```python
from build123d import *

# Parameters (mm, degrees)
SKETCH_1_R      = 15
SKETCH_1_R_2    = 1
EXTRUDE_1_DEPTH = 2
EXTRUDE_2_DEPTH = 1
SKETCH_4_R      = 10.5
SKETCH_4_R_2    = 0.75
EXTRUDE_3_DEPTH = 2
SKETCH_5_R      = 10.5
SKETCH_5_R_2    = 0.75
EXTRUDE_4_DEPTH = 2
EXTRUDE_5_DEPTH = 1
SKETCH_7_R      = 10.5
SKETCH_7_R_2    = 0.75
EXTRUDE_6_DEPTH = 2
SKETCH_8_R      = 10.5
SKETCH_8_R_2    = 0.75
EXTRUDE_7_DEPTH = 2


with BuildPart() as part:
    # 草图1 → 凸台-拉伸1 (new body)
    with BuildSketch(Plane(origin=(0, 0, 0), x_dir=(1, 0, 0), z_dir=(0, 1, 0))):
        with Locations(Location((0, 0, 0), (0, 0, 270))):
            Circle(SKETCH_1_R)
        with Locations(Location((7.778174593, 7.778174593, 0), (0, 0, 270))):
            Circle(SKETCH_1_R_2, mode=Mode.SUBTRACT)
        with Locations(Location((-7.778174593, 7.778174593, 0), (0, 0, 270))):
            Circle(SKETCH_1_R_2, mode=Mode.SUBTRACT)
        with Locations(Location((-7.778174593, -7.778174593, 0), (0, 0, 270))):
            Circle(SKETCH_1_R_2, mode=Mode.SUBTRACT)
        with Locations(Location((7.778174593, -7.778174593, 0), (0, 0, 270))):
            Circle(SKETCH_1_R_2, mode=Mode.SUBTRACT)
    extrude(amount=EXTRUDE_1_DEPTH)

    # 草图2 → 旋转1 (revolve)
    with BuildSketch(Plane(origin=(0, 0, 0), x_dir=(0, 0, -1), z_dir=(1, 0, 0))):
        with BuildLine():
            Line((0, 2), (0, 7))
            ThreePointArc((0, 7), (3.535533906, 5.535533906), (5, 2))
            Line((5, 2), (0, 2))
        make_face()
    revolve(axis=Axis((0, 2, 0), (0, 1, 0)))

    # 草图3 → 凸台-拉伸2 (add, symmetric)
    with BuildSketch(Plane.XY):
        Polygon((0, 2), (24.148145657, 8.470476128), (16.420739047, 8.470476128), (0, 4.070552361), (0, 4.828427125), (-28.991378029, 33.819805153), (-31.819805153, 33.819805153), align=None)
    extrude(amount=EXTRUDE_2_DEPTH, both=True)

    # 草图4 → 凸台-拉伸3 (add)
    with BuildSketch(Plane(origin=(0, 8.470476128, 0), x_dir=(1, 0, 0), z_dir=(0, 1, 0))):
        with Locations(Location((29.148145657, 0, 0), (0, 0, 174.5349762))):
            Circle(SKETCH_4_R)
        with Locations(Location((29.148145657, 0, 0), (0, 0, 270))):
            Circle(SKETCH_4_R_2, mode=Mode.SUBTRACT)
    extrude(amount=EXTRUDE_3_DEPTH)

    # 草图5 → 凸台-拉伸4 (add)
    with BuildSketch(Plane(origin=(0, 33.819805153, 0), x_dir=(1, 0, 0), z_dir=(0, 1, 0))):
        with Locations(Location((-36.819805153, 0, 0), (0, 0, 270))):
            Circle(SKETCH_5_R)
        with Locations(Location((-36.819805153, 0, 0), (0, 0, 270))):
            Circle(SKETCH_5_R_2, mode=Mode.SUBTRACT)
    extrude(amount=EXTRUDE_4_DEPTH)

    # 草图6 → 凸台-拉伸5 (add, symmetric)
    with BuildSketch(Plane(origin=(0, 0, 0), x_dir=(0, 0, -1), z_dir=(1, 0, 0))):
        Polygon((0, 2), (30.310889132, 19.5), (26.310889132, 19.5), (0, 4.309401077), (0, 6), (-20.190598923, 40.97114317), (-22.5, 40.97114317), align=None)
    extrude(amount=EXTRUDE_5_DEPTH, both=True)

    # 草图7 → 凸台-拉伸6 (add)
    with BuildSketch(Plane(origin=(0, 19.5, 0), x_dir=(1, 0, 0), z_dir=(0, 1, 0))):
        with Locations(Location((0, 35.310889132, 0), (0, 0, 270))):
            Circle(SKETCH_7_R)
        with Locations(Location((0, 35.310889132, 0), (0, 0, 270))):
            Circle(SKETCH_7_R_2, mode=Mode.SUBTRACT)
    extrude(amount=EXTRUDE_6_DEPTH)

    # 草图8 → 凸台-拉伸7 (add)
    with BuildSketch(Plane(origin=(0, 40.97114317, 0), x_dir=(1, 0, 0), z_dir=(0, 1, 0))):
        with Locations(Location((0, -27.5, 0), (0, 0, 270))):
            Circle(SKETCH_8_R)
        with Locations(Location((0, -27.5, 0), (0, 0, 270))):
            Circle(SKETCH_8_R_2, mode=Mode.SUBTRACT)
    extrude(amount=EXTRUDE_7_DEPTH)


solid = part.part
```
Work out the finished part from the listing and answer in its coordinate system (mm). A direction names the side the tool comes from. Give positions to 0.01 mm unless a question says otherwise; leave off trailing zeros. Write each loop counter-clockwise with the first axis right and the second up, starting at its lowest first coordinate (ties: lowest second). Pieces come first, ordered by that corner, then holes.
(1) The part is cut by section D-D on x = 33. Write down the section's boundary in (y, z), plus the area to 3 significant figures.
Final values:
outline: (8.47, -9.77) - (10.47, -9.77) - (10.47, 9.77) - (8.47, 9.77) - close
area: 39.1 mm2
(2) The part is cut by section B-B on y = 32.5. Write down the section's boundary in (x, z), plus the area to 3 significant figures.
Final values:
outline: (-30.5, -1) - (-27.67, -1) - (-27.67, 1) - (-30.5, 1) - close; (-1, 15.3) - (1, 15.3) - (1, 17.61) - (-1, 17.61) - close
area: 10.3 mm2
(3) Flat-ended cylindrical pins translate along their axes: pin 1 Ø8 at (y, z) = (16.5, -18.5) entering from -X; pin 2 Ø2 at (x, z) = (-8.5, -32) entering from +Y; pin 3 Ø23 at (x, z) = (-38, -2.5) entering from +Y; pin 4 Ø2.5 at (x, z) = (-7.78, 7.78) entering from -Y. Find the tip coordinate at first contact, or state that the pin passes through.
Final values:
pin 1: stops at x = -1
pin 2: stops at y = 21.5
pin 3: stops at y = 35.82
pin 4: stops at y = 0
(4) The part is cut by section C-C on z = 13. Write down the section's boundary in (x, y), plus the area to 3 significant figures.
Final values:
outline: (-7.48, 0) - (7.48, 0) - (7.48, 2) - (-7.48, 2) - close; (-1, 24.52) - (1, 24.52) - (1, 28.52) - (-1, 28.52) - close
area: 37.9 mm2
(5) The part is cut by section A-A on y = 16.5. Write down the section's boundary in (x, z), plus the area to 3 significant figures.
Final values:
outline: (-14.5, -1) - (-11.67, -1) - (-11.67, 1) - (-14.5, 1) - close; (-1, -25.11) - (1, -25.11) - (1, -21.11) - (-1, -21.11) - close; (-1, 6.06) - (1, 6.06) - (1, 8.37) - (-1, 8.37) - close
area: 18.3 mm2
(6) Straight lines are drawn through the part: line 1 (X direction, y = 35.25, z = 0); line 2 (Y direction, x = 12.5, z = -2); line 3 (Y direction, x = -38.5, z = -2). For each, find the intervals that lie inside material, in ascending order.
Final values:
line 1: x = -47.32 to -37.57, -36.07 to -26.32
line 2: y = 0 to 2
line 3: y = 33.82 to 35.82
(7) The mould has two halves that part along Y. Classify faces 5 (the flat face through (0.014, 23.85, 12.615)), 6 (the cylindrical face through (0.66, 0.986, -14.985)), 7 (the flat face through (30, 8.47, -2)): pulls with the +Y half, pulls with the -Y half, needs draft (parallel to the pull), parting line crosses it, or undercut.
Final values:
face 5: undercut
face 6: needs draft
face 7: pulls with the -Y half
(8) Which of the six approach directions +Z, -Z, +X, -X, +Y, -Y give full straight-line access (tool end or side, diameter ignored) to faces 1 (the flat face through (-18, 20, 0)), 2 (the flat face through (27, 10.47, 0)), 3 (the flat face through (14.3, 5.83, 0.01)), 4 (the flat face through (10.2, 6.804, 0.014))?
Final values:
face 1: +Z, -Z, -X
face 2: +Z, -Z, +X, +Y
face 3: +Z, -Z, +X
face 4: +Z, -Z, +Y
